from build123d import *

# Parameters (mm, degrees)
SKETCH1_W                          = 95.25
SKETCH1_H                          = 95.25
BASE_EXTRUDE_DEPTH                 = 2.54
F_3_16_0_1875_DIAMETER_HOLE1_D     = 4.7625
F_3_16_0_1875_DIAMETER_HOLE1_DEPTH = 2.54
F_3_16_0_1875_DIAMETER_HOLE1_TIP   = 1.430799349
CUT_EXTRUDE1_REACH                 = 69.4
F_5_16_0_3125_DIAMETER_HOLE1_D     = 7.9375
CHAMFER1_SIZE                      = 1.905


with BuildPart() as part:
    # Sketch1 → Base Extrude (new body)
    with BuildSketch(Plane(origin=(0, 0, 0), x_dir=(1, 0, 0), z_dir=(0, 1, 0))):
        Rectangle(SKETCH1_W, SKETCH1_H)
    extrude(amount=BASE_EXTRUDE_DEPTH)

    # 3/16 (0.1875) Diameter Hole1
    with Locations(Plane(origin=(0, 2.54, 0), x_dir=(1, 0, 0), z_dir=(0, 1, 0))):
        with Locations((-42.207203769, 42.207203769), (42.207203769, 42.207203769), (42.207203769, -42.207203769), (-42.207203769, -42.207203769)):
            Hole(F_3_16_0_1875_DIAMETER_HOLE1_D / 2, depth=F_3_16_0_1875_DIAMETER_HOLE1_DEPTH)
            with Locations((0, 0, -(F_3_16_0_1875_DIAMETER_HOLE1_DEPTH + F_3_16_0_1875_DIAMETER_HOLE1_TIP / 2))):  # 118° drill point
                Cone(0, F_3_16_0_1875_DIAMETER_HOLE1_D / 2, F_3_16_0_1875_DIAMETER_HOLE1_TIP, mode=Mode.SUBTRACT)

    # Sketch12 → Cut-Extrude1 (cut, up to next)
    with BuildSketch(Plane(origin=(0, 2.54, 0), x_dir=(1, 0, 0), z_dir=(0, 1, 0)), mode=Mode.PRIVATE) as cut_extrude1_sk1:
        Polygon((-15.006272328, 8.830810905), (-15.006272328, -8.830810905), (-47.625, -30.869032315), (-47.625, 30.869032315), align=None)
    cut_extrude1_tool1 = extrude(cut_extrude1_sk1.sketch, amount=-CUT_EXTRUDE1_REACH, mode=Mode.PRIVATE) & part.part
    # Sketch12 → Cut-Extrude1 (cut, up to next)
    with BuildSketch(Plane(origin=(0, 2.54, 0), x_dir=(1, 0, 0), z_dir=(0, 1, 0)), mode=Mode.PRIVATE) as cut_extrude1_sk2:
        Polygon((30.869032315, 47.625), (-30.869032315, 47.625), (-8.830810905, 15.006272328), (8.830810905, 15.006272328), align=None)
    cut_extrude1_tool2 = extrude(cut_extrude1_sk2.sketch, amount=-CUT_EXTRUDE1_REACH, mode=Mode.PRIVATE) & part.part
    # Sketch12 → Cut-Extrude1 (cut, up to next)
    with BuildSketch(Plane(origin=(0, 2.54, 0), x_dir=(1, 0, 0), z_dir=(0, 1, 0)), mode=Mode.PRIVATE) as cut_extrude1_sk3:
        Polygon((47.625, -30.869032315), (47.625, 30.869032315), (15.006272328, 8.830810905), (15.006272328, -8.830810905), align=None)
    cut_extrude1_tool3 = extrude(cut_extrude1_sk3.sketch, amount=-CUT_EXTRUDE1_REACH, mode=Mode.PRIVATE) & part.part
    # Sketch12 → Cut-Extrude1 (cut, up to next)
    with BuildSketch(Plane(origin=(0, 2.54, 0), x_dir=(1, 0, 0), z_dir=(0, 1, 0)), mode=Mode.PRIVATE) as cut_extrude1_sk4:
        Polygon((-30.869032315, -47.625), (30.869032315, -47.625), (8.830810905, -15.006272328), (-8.830810905, -15.006272328), align=None)
    cut_extrude1_tool4 = extrude(cut_extrude1_sk4.sketch, amount=-CUT_EXTRUDE1_REACH, mode=Mode.PRIVATE) & part.part
    add(cut_extrude1_tool1.solids().sort_by_distance((-34.333527, 2.54, 0))[0], mode=Mode.SUBTRACT)
    add(cut_extrude1_tool2.solids().sort_by_distance((0, 2.54, -34.333527))[0], mode=Mode.SUBTRACT)
    add(cut_extrude1_tool3.solids().sort_by_distance((34.333527, 2.54, 0))[0], mode=Mode.SUBTRACT)
    add(cut_extrude1_tool4.solids().sort_by_distance((0, 2.54, 34.333527))[0], mode=Mode.SUBTRACT)

    # 5/16 (0.3125) Diameter Hole1 (through all)
    with Locations(Plane(origin=(0, 2.54, 0), x_dir=(1, 0, 0), z_dir=(0, 1, 0))):
        with Locations((0, 0)):
            Hole(F_5_16_0_3125_DIAMETER_HOLE1_D / 2)

    # Chamfer1
    chamfer1_edges = [part.edges().sort_by_distance(p)[0] for p in [
        (-39.825953769, 2.54, 42.207203769),
        (44.588453769, 2.54, 42.207203769),
        (44.588453769, 2.54, -42.207203769),
        (-39.825953769, 2.54, -42.207203769),
    ]]
    chamfer(chamfer1_edges, length=CHAMFER1_SIZE)


solid = part.part
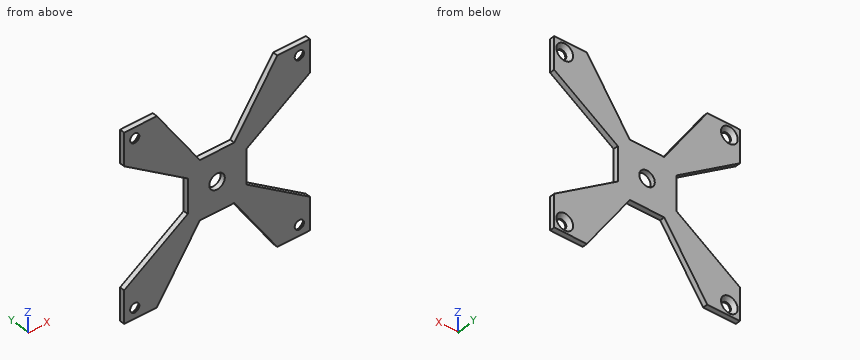
For this review, take the finished solid that the model builds, in its own axes (mm). Give positions to 0.01 mm unless a question says otherwise; leave off trailing zeros. Loops run counter-clockwise (first coordinate to the right, second up) from the corner with the lowest first, then second, coordinate; pieces in that order, holes last. Notation, with made-up numbers: (8.25, 60) - (45.25, 60) arc R31 cw to (45.25, 96) - close; hole circle Ø2 at (51, 4.5). An arc over 180 degrees is marked (long way). Write each question's results on one line, items separated by ' | '.
(1) For pin 1 Ø1.5 at (x, y) = (-14.5, 1) entering from +Z; pin 2 Ø6 at (x, z) = (-42.21, -42.21) entering from +Y; pin 3 Ø4 at (x, z) = (-42.21, 42.21) entering from +Y; pin 4 Ø1.3 at (x, y) = (-0.5, 1.5) entering from +Z, all flat-tipped, find the tip position at first contact; note any pin that passes through.
Conclusion:
pin 1: z = 24.51 | pin 2: y = 1.26 | pin 3: through | pin 4: z = 15.01
(2) Take a section at B-B (z = 0). Give the boundary of the cut face in (x, y), then the cut area to 3 significant figures.
Conclusion:
outline: (-15.01, 0) - (-3.97, 0) - (-3.97, 2.54) - (-15.01, 2.54) - close; (3.97, 0) - (15.01, 0) - (15.01, 2.54) - (3.97, 2.54) - close | area: 56.1 mm^2
(3) Take a section at C-C (y = 1.8). Give the boundary of the cut face in (x, z) (1 decimal).
Conclusion:
outline: (-47.6, -47.6) - (-30.9, -47.6) - (-8.8, -15) - (8.8, -15) - (30.9, -47.6) - (47.6, -47.6) - (47.6, -30.9) - (15, -8.8) - (15, 8.8) - (47.6, 30.9) - (47.6, 47.6) - (30.9, 47.6) - (8.8, 15) - (-8.8, 15) - (-30.9, 47.6) - (-47.6, 47.6) - (-47.6, 30.9) - (-15, 8.8) - (-15, -8.8) - (-47.6, -30.9) - close; hole circle Ø7.1 at (-42.2, -42.2); hole circle Ø7.1 at (-42.2, 42.2); hole circle Ø7.9 at (0, 0); hole circle Ø7.1 at (42.2, -42.2); hole circle Ø7.1 at (42.2, 42.2)
(4) Take a section at A-A (x = 0). Give the boundary of the cut face in (y, z).
Conclusion:
outline: (0, -15.01) - (2.54, -15.01) - (2.54, -3.97) - (0, -3.97) - close; (0, 3.97) - (2.54, 3.97) - (2.54, 15.01) - (0, 15.01) - close
(5) Take a section at D-D (x = -12.5). Give the boundary of the cut face in (y, z).
Conclusion:
outline: (0, -20.44) - (2.54, -20.44) - (2.54, 20.44) - (0, 20.44) - close
(6) For line 1 along Z through (x, y) = (0, 0.8); line 2 along Z through (x, y) = (29, 2.2); line 3 along X through (y, z) = (1, 37) (3 decimals), list the stretches that pass through material, from the lowest coordinate up.
Conclusion:
line 1: -15.01 to -3.97, 3.97 to 15.01 | line 2: -44.86 to -18.29, 18.29 to 44.86 | line 3: -47.625 to -23.69, 23.69 to 47.625
